Part model, mm, in its own coordinate system. Face numbers are marked on the shaded views. Coordinates: 2 decimals unless noted, no trailing zeros. Loops run counter-clockwise (first coordinate to the right, second up) from the corner with the lowest first, then second, coordinate; pieces in that order, holes last. Notation, with made-up numbers: M 66,6 L 101,6 A18 ccw 101,15 Z; hole C -38,46 d7. An arc over 180 degrees is marked long. Use CSV: the item, a comma, the result in double quotes. Start each with the question number.
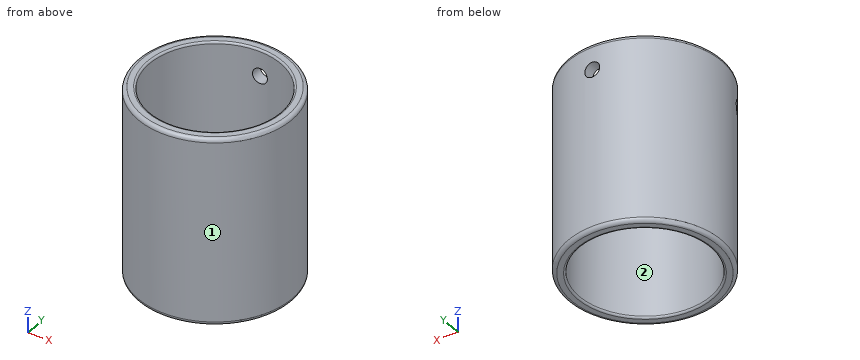
from build123d import *

# Parameters (mm, degrees)
BOSS_EXTRUDE1_DEPTH      = 30
BOSS_EXTRUDE1_DEPTH_BACK = 20
SKETCH1_R                = 20.5
SKETCH1_R_2              = 17.5
SKETCH3_R                = 2
CUT_EXTRUDE1_DEPTH       = 42.71930009
CIRPATTERN1_COUNT        = 2
CIRPATTERN1_ANGLE        = 120
FILLET1_R                = 1
FILLET2_R                = 0.5


with BuildPart() as part:
    # Sketch1 → Boss-Extrude1 (new, two sides: drawn at the far end of the back side and taken through both)
    with BuildSketch(Plane.XY.offset(-BOSS_EXTRUDE1_DEPTH_BACK)):
        Circle(SKETCH1_R)
        Circle(SKETCH1_R_2, mode=Mode.SUBTRACT)
    extrude(amount=BOSS_EXTRUDE1_DEPTH + BOSS_EXTRUDE1_DEPTH_BACK)

    # Sketch3 → Cut-Extrude1 (cut, through all)
    with BuildSketch(Plane(origin=(0, 0, 0), x_dir=(1, 0, 0), z_dir=(0, 1, 0))):
        with Locations(Location((0, -23, 0), (0, 0, 90))):
            Circle(SKETCH3_R)
    cut_extrude1 = extrude(amount=CUT_EXTRUDE1_DEPTH, mode=Mode.SUBTRACT)

    # CirPattern1: Cut-Extrude1 ×2 about axis
    cirpattern1_axis = Axis((0, 0, -20), (0, 0, 1))
    for i in range(1, CIRPATTERN1_COUNT):
        add(cut_extrude1.rotate(cirpattern1_axis, i * CIRPATTERN1_ANGLE / (CIRPATTERN1_COUNT - 1)), mode=Mode.SUBTRACT)

    # Fillet1
    fillet1_edges = [part.edges().sort_by_distance(p)[0] for p in [
        (-20.5, 0, -20),
        (-20.5, 0, 30),
    ]]
    fillet(fillet1_edges, radius=FILLET1_R)

    # Fillet2
    fillet2_edges = [part.edges().sort_by_distance(p)[0] for p in [
        (-17.5, 0, -20),
        (-17.5, 0, 30),
    ]]
    fillet(fillet2_edges, radius=FILLET2_R)


solid = part.part
1. Slice it at C-C, the plane z = -0.5. List the corners of the cut face in (x, y), and give its area (3 significant figures).
2. Two-plate mould, pull along X, no slides. Class the marked faces 1 and 2: pulls with the +X half, pulls with the -X half, needs draft (parallel to the pull), parting line crosses it, or undercut.
3. Slice it at B-B, the plane z = 23. List the corners of the cut face in (x, y), and give its area (3 significant figures).
4. Wall check: probe 1 along Y at (x, z) = (0, -4); probe 2 along Y at (x, z) = (-1.5, 11); probe 3 along X at (y, z) = (18.35, 23). Give the ranges that are in metal, low to high.
5. Pin check, flat tips, straight feed: pin 1 (3.5 mm diameter, centred on x = 0, z = 23, fed in from +Y); pin 2 (3 mm diameter, centred on y = -10, z = -8.5, fed in from -X); pin 3 (1.5 mm diameter, centred on x = -5, z = 1.5, fed in from -Y). Stop position of each tip, or through.
6. Slice it at A-A, the plane y = 0. List the corners of the cut face in (x, z).
Found:
1,outline,"C 0,0 d41; hole C 0,0 d35"
1,area,"358 mm^2"
2,face 1,"parting line crosses it"
2,face 2,"undercut"
3,outline,"M -18.67,-8.47 L -16.06,-6.96 A17.5 cw -2,17.39 L -2,20.4 A20.5 ccw Z; M -16.67,-11.93 A20.5 ccw long 2,20.4 L 2,17.39 A17.5 cw long -14.06,-10.42 Z"
3,area,"334 mm^2"
4,probe 1,"-20.5 to -17.5, 17.5 to 20.5"
4,probe 2,"-20.45 to -17.44, 17.44 to 20.45"
4,probe 3,"-9.14 to -2, 2 to 9.14"
5,pin 1,"y = -17.41"
5,pin 2,"x = -18.65"
5,pin 3,"y = -20.05"
6,outline,"M -20.5,-19 A1 ccw -19.5,-20 L -18,-20 A0.5 ccw -17.5,-19.5 L -17.5,29.5 A0.5 ccw -18,30 L -19.5,30 A1 ccw -20.5,29 Z; M 17.5,-19.5 A0.5 ccw 18,-20 L 19.5,-20 A1 ccw 20.5,-19 L 20.5,29 A1 ccw 19.5,30 L 18,30 A0.5 ccw 17.5,29.5 Z"
